from build123d import *

# Parameters (mm, degrees)
SKETCH_1_R          = 1.1
EXTRUDE_1_DEPTH     = 3
SKETCH_2_W          = 35
SKETCH_2_H          = 11
EXTRUDE_2_DEPTH     = 3
FILLET_1_R          = 1.5
SKETCH_3_R          = 1.5
CUT_EXTRUDE_1_DEPTH = 3
FILLET_2_R          = 2


with BuildPart() as part:
    # 草图1 → 凸台-拉伸1 (new body)
    with BuildSketch(Plane.XY):
        with BuildLine():
            Line((-13.25, -3.875), (-13.25, -2.625))
            Line((-13.25, -2.625), (-15.25, -0.625))
            ThreePointArc((-15.25, -0.625), (-16.840990258, 0.034009742), (-17.5, 1.625))
            Line((-17.5, 1.625), (-17.5, 8.625))
            Line((-17.5, 8.625), (-13.25, 8.625))
            Line((-13.25, 8.625), (13.25, 8.625))
            Line((13.25, 8.625), (17.5, 8.625))
            Line((17.5, 8.625), (17.5, 1.625))
            ThreePointArc((17.5, 1.625), (16.840990258, 0.034009742), (15.25, -0.625))
            Line((15.25, -0.625), (13.25, -2.625))
            Line((13.25, -2.625), (13.25, -3.875))
            ThreePointArc((13.25, -3.875), (12.00520382, -6.88020382), (9, -8.125))
            Line((9, -8.125), (9, -10.125))
            Line((9, -10.125), (-9, -10.125))
            Line((-9, -10.125), (-9, -8.125))
            ThreePointArc((-9, -8.125), (-12.00520382, -6.88020382), (-13.25, -3.875))
        make_face()
        with Locations((-15.25, 1.625)):
            Circle(SKETCH_1_R, mode=Mode.SUBTRACT)
        with Locations((15.25, 1.625)):
            Circle(SKETCH_1_R, mode=Mode.SUBTRACT)
    extrude(amount=EXTRUDE_1_DEPTH)

    # 草图2 → 凸台-拉伸2 (add)
    with BuildSketch(Plane(origin=(0, 8.625, 0), x_dir=(1, 0, 0), z_dir=(0, 1, 0))):
        with Locations((0, -5.5)):
            Rectangle(SKETCH_2_W, SKETCH_2_H)
    extrude(amount=EXTRUDE_2_DEPTH)

    # 圆角1
    fillet_1_edges = [part.edges().sort_by_distance(p)[0] for p in [
        (0, 8.625, 3),
        (0, 11.625, 0),
    ]]
    fillet(fillet_1_edges, radius=FILLET_1_R)

    # 草图3 → 切除-拉伸1 (cut)
    with BuildSketch(Plane.XZ.offset(-8.625)):
        with Locations(Location((13.5, 7.75, 0), (0, 0, 270))):
            Circle(SKETCH_3_R)
        with Locations(Location((-13.5, 7.75, 0), (0, 0, 270))):
            Circle(SKETCH_3_R)
    extrude(amount=-CUT_EXTRUDE_1_DEPTH, mode=Mode.SUBTRACT)

    # 圆角2
    fillet_2_edges = [part.edges().sort_by_distance(p)[0] for p in [
        (9, -10.125, 1.5),
        (-9, -10.125, 1.5),
    ]]
    fillet(fillet_2_edges, radius=FILLET_2_R - 0.0001)  # a hair under: the kernel refuses the full size


solid = part.part
Build history of the part. All positions in model axes, mm. A direction names the side the tool comes from. Coordinates: 2 decimals unless noted, no trailing zeros. Write each loop counter-clockwise with the first axis right and the second up, starting at its lowest first coordinate (ties: lowest second). Pieces come first, ordered by that corner, then holes.
(1) 3-axis set-ups, long thin cutter, end or side, ignore diameter. For faces 4 (the flat face through (0, 8.625, 8)), 5 (the flat face through (-13.25, -3, 1)), 6 (the cylindrical face through (12.038, -6.847, 1.479)): which of +Z, -Z, +X, -X, +Y, -Y reach the whole face in a straight line?
(2) Cut at D-D on z = 9.75. List the corners of the cut face in (x, y) (3 decimals), and give its area (3 significant figures).
(3) Cut at A-A on z = 7.75. List the corners of the cut face in (x, y) (3 decimals).
(4) Cut at B-B on x = 14.5. List the corners of the cut face in (y, z) (3 decimals).
(5) Mould opens along X. For faces 1 (the cylindrical face through (0.245, 11.174, 0.428)), 2 (the flat face through (14.264, -1.611, 1.479)), 3 (the cylindrical face through (-16.35, 1.67, 1.48)) say: pulls with the +X half, pulls with the -X half, needs draft (parallel to the pull), parting line crosses it, or undercut.
(6) Drill centre lines: line 1 (X direction, y = 1.5, z = 1); line 2 (X direction, y = 10.6, z = 7.75); line 3 (Y direction, x = 15.25, z = 2.3) (3 decimals). Where is each one in solid material? Low to high.
(7) Cut at C-C on x = 4. List the corners of the cut face in (y, z) (3 decimals).
(8) Pin check, flat tips, straight feed: pin 1 Ø1.5 at (x, z) = (-10.5, 8.5) entering from -Y (3 decimals); pin 2 Ø1.5 at (x, y) = (-2.5, -3.5) entering from +Z; pin 3 Ø1 at (y, z) = (-3, 1.5) entering from +X (3 decimals). Stop position of each tip, or through.
Working result:
1. face 4: +Z, +X, -X, -Y
1. face 5: +Z, -Z, -X, -Y
1. face 6: +Z, -Z, +X, -Y
2. outline: (-17.5, 8.625) - (17.5, 8.625) - (17.5, 11.625) - (-17.5, 11.625) - close
2. area: 105 mm2
3. outline: (-17.5, 8.625) - (-15, 8.625) - (-15, 11.625) - (-17.5, 11.625) - close; (-12, 8.625) - (12, 8.625) - (12, 11.625) - (-12, 11.625) - close; (15, 8.625) - (17.5, 8.625) - (17.5, 11.625) - (15, 11.625) - close
4. outline: (-1.375, 0) - (0.82, 0) - (0.82, 3) - (-1.375, 3) - close; (2.43, 0) - (10.125, 0) arc R1.5 ccw to (11.625, 1.5) - (11.625, 6.632) - (8.625, 6.632) - (8.625, 4.5) arc R1.5 cw to (7.125, 3) - (2.43, 3) - close; (8.625, 8.868) - (11.625, 8.868) - (11.625, 11) - (8.625, 11) - close
5. face 1: needs draft
5. face 2: pulls with the +X half
5. face 3: undercut
6. line 1: x = -17.5 to -16.34, -14.16 to 14.16, 16.34 to 17.5
6. line 2: x = -17.5 to -15, -12 to 12, 15 to 17.5
6. line 3: y = -0.625 to 0.525, 2.725 to 11.625
7. outline: (-10.125, 0) - (10.125, 0) arc R1.5 ccw to (11.625, 1.5) - (11.625, 11) - (8.625, 11) - (8.625, 4.5) arc R1.5 cw to (7.125, 3) - (-10.125, 3) - close
8. pin 1: stops at y = 8.625
8. pin 2: stops at z = 3
8. pin 3: stops at x = 13.375
